Work out the finished part from the listing and answer in its coordinate system (mm). Give positions to 0.01 mm unless a question says otherwise; leave off trailing zeros. Order: outer loops, then holes, each group sorted by start corner. A loop starts at its lowest first (then second) coordinate and runs counter-clockwise, first axis right, second up.
```python
from build123d import *

# Parameters (mm, degrees)
SKETCH1_W           = 342.9
SKETCH1_H           = 342.9
BOSS_EXTRUDE1_DEPTH = 8.5
SKETCH2_R           = 4
CUT_EXTRUDE1_DEPTH  = 243.615858921
SKETCH3_R           = 7.5
SKETCH3_R_2         = 5.15
CUT_EXTRUDE3_DEPTH  = 10


with BuildPart() as part:
    # Sketch1 → Boss-Extrude1 (new body)
    with BuildSketch(Plane(origin=(0, 0, 0), x_dir=(1, 0, 0), z_dir=(0, 1, 0))):
        Rectangle(SKETCH1_W, SKETCH1_H)
    extrude(amount=BOSS_EXTRUDE1_DEPTH)

    # Sketch2 → Cut-Extrude1 (cut, through all)
    with BuildSketch(Plane(origin=(0, 8.5, 0), x_dir=(1, 0, 0), z_dir=(0, 1, 0))):
        with Locations(Location((-158.225, 158.225, 0), (0, 0, 270))):
            Circle(SKETCH2_R)
        with Locations(Location((-158.225, 0, 0), (0, 0, 270))):
            Circle(SKETCH2_R)
        with Locations(Location((-158.225, -158.225, 0), (0, 0, 270))):
            Circle(SKETCH2_R)
        with Locations(Location((158.225, 158.225, 0), (0, 0, 270))):
            Circle(SKETCH2_R)
        with Locations(Location((158.225, 0, 0), (0, 0, 270))):
            Circle(SKETCH2_R)
        with Locations(Location((158.225, -158.225, 0), (0, 0, 270))):
            Circle(SKETCH2_R)
    extrude(amount=-CUT_EXTRUDE1_DEPTH, mode=Mode.SUBTRACT)

    # Sketch3 → Cut-Extrude3 (cut)
    with BuildSketch(Plane(origin=(0, 8.5, 0), x_dir=(1, 0, 0), z_dir=(0, 1, 0))):
        with Locations(Location((-158.225, 158.225, 0), (0, 0, 270))):
            Circle(SKETCH3_R)
        with Locations(Location((-158.225, -158.225, 0), (0, 0, 270))):
            Circle(SKETCH3_R)
        with Locations(Location((-158.225, 0, 0), (0, 0, 270))):
            Circle(SKETCH3_R_2)
        with Locations(Location((158.225, 0, 0), (0, 0, 270))):
            Circle(SKETCH3_R)
        with Locations(Location((158.225, 158.225, 0), (0, 0, 270))):
            Circle(SKETCH3_R_2)
        with Locations(Location((158.225, -158.225, 0), (0, 0, 270))):
            Circle(SKETCH3_R_2)
    extrude(amount=-CUT_EXTRUDE3_DEPTH, mode=Mode.SUBTRACT)


solid = part.part
```
1. A straight line is drawn through the part: probe 1 along X at (y, z) = (3, 0) (3 decimals). Find the intervals that lie inside material, in ascending order.
Findings below:
probe 1: x = -171.45 to -163.375, -153.075 to 150.725, 165.725 to 171.45
2. The part is cut by section A-A (z = 0). Write down the section's boundary in (x, y) (3 decimals), then the cut area to 3 significant figures.
Findings below:
outline: (-171.45, 0) - (-163.375, 0) - (-163.375, 8.5) - (-171.45, 8.5) - close; (-153.075, 0) - (150.725, 0) - (150.725, 8.5) - (-153.075, 8.5) - close; (165.725, 0) - (171.45, 0) - (171.45, 8.5) - (165.725, 8.5) - close
area: 2,700 mm2
3. Given P1, Ø6, axis at x = 74, z = 71, coming from the -Y side, flat-ended and moving along its own axis, determine where the tip first touches the part or whether it passes through.
Findings below:
P1: stops at y = 0
4. The mould has two halves that part along Z. Classify faces 1 (the face through (-2, 4, 171.45)), 2 (the face through (-2, 8.5, -2)), 3 (the face through (153.656, 4.31, -155.849)): pulls with the +Z half, pulls with the -Z half, needs draft (parallel to the pull), parting line crosses it, or undercut.
Findings below:
face 1: pulls with the +Z half
face 2: needs draft
face 3: undercut
